from build123d import *

# Parameters (mm, degrees)
F0_R          = 5
F1_ANGLE_BACK = 60
F1_ANGLE      = 120
F2_W          = 25.9252840082
F2_H          = 11.7293265872
F3_DEPTH      = 25
F3_DEPTH_BACK = 25
F4_W          = 50
F4_H          = 15
F5_DEPTH      = 100
F6_R          = 5


# Not quite as in the source:
# - a feature of the source that left no trace in its solid (it failed there, or was rolled back) is left out


with BuildPart() as f1:
    # F0 (on Right) → F1 (revolve)
    with BuildSketch(Plane.YZ, mode=Mode.PRIVATE) as f1_sk:
        with Locations((30.3885055535, 0)):
            Circle(F0_R)
    revolve(f1_sk.sketch.rotate(Axis((0, -119.6114944465, -16.3725827584), (0, 0, -1)), -F1_ANGLE_BACK), axis=Axis((0, -119.6114944465, -16.3725827584), (0, 0, -1)), revolution_arc=F1_ANGLE)

    # F2 (on Right) → F3 (join, two sides)
    with BuildSketch(Plane.YZ) as f3_sk:
        with Locations((37.9626420041, -4.1353367064)):
            Rectangle(F2_W, F2_H)
    extrude(amount=F3_DEPTH)
    extrude(f3_sk.sketch, amount=-F3_DEPTH_BACK)

    # F4 (on face) → F5 (join)
    with BuildSketch(Plane.XY.offset(1.7293265872)):
        with Locations((0, 43.4252840082)):
            Rectangle(F4_W, F4_H)
    extrude(amount=F5_DEPTH)

    # F6
    f6_edges = [f1.edges().sort_by_distance(p)[0] for p in [
        (0, 50.925284, -10),
        (25, 50.925284, 45.864663),
        (0, 50.925284, 101.729327),
        (-25, 50.925284, 45.864663),
    ]]
    fillet(f6_edges, radius=F6_R)


solid = f1.part
Could you check a few things on this model? Use its own coordinates, in mm. Coordinates: 2 decimals unless noted, no trailing zeros. Write each loop counter-clockwise with the first axis right and the second up, starting at its lowest first coordinate (ties: lowest second). Pieces come first, ordered by that corner, then holes. Notation, with made-up numbers: (-1, 73) - (51, 73) arc R11 cw to (51, 78) - close; hole circle Ø4 at (11, -21). An arc over 180 degrees is marked (long way). Write item = value, one per line.
1) We'd pull the mould along X, two halves only. Please class faces 1 (the flat face through (0, 25, -6)), 2 (the cylindrical face through (0.35, 49.499, 100.226)), 3 (the flat face through (129.84, -44.65, 0.07)), 4 (the flat face through (-129.84, -44.65, 0.07)): +X half, -X half, draft (parallel to the pull), parting line (faces both ways), or undercut.
Result set:
face_1 = undercut
face_2 = draft
face_3 = +X half
face_4 = -X half
2) Suppose I cut it at A-A on z = 8. Please give me the cut outline in (x, y), plus the area to 3 significant figures.
Result set:
outline = (-25, 35.93) - (25, 35.93) - (25, 45.93) arc R5 ccw to (20, 50.93) - (-20, 50.93) arc R5 ccw to (-25, 45.93) - close
area = 739 mm2
3) Will these pins go through, and if not, where does the flat tip stop? pin 1 Ø0.9 at (x, y) = (-10.5, 35) entering from +Z; pin 2 Ø6.5 at (y, z) = (34.5, 51) entering from +X; pin 3 Ø10.5 at (y, z) = (36.5, 66) entering from -X.
Result set:
pin_1 = 2.14
pin_2 = 25
pin_3 = -25
4) Please list where these lines run through material, in increasing order: line 1 (Z direction, x = -14, y = 29); line 2 (X direction, y = 36, z = -1.5); line 3 (Z direction, x = -81.5, y = 1). Write a range as [from, to].
Result set:
line_1 = [-10, 4.95]
line_2 = [-25, 25]
line_3 = [-2.31, 2.31]
5) Suppose I cut it at B-B on y = 39.5. Please give me the cut outline in (x, z), plus the area to 3 significant figures.
Result set:
outline = (-25, -10) - (25, -10) - (25, 101.73) - (-25, 101.73) - close
area = 5,590 mm2
